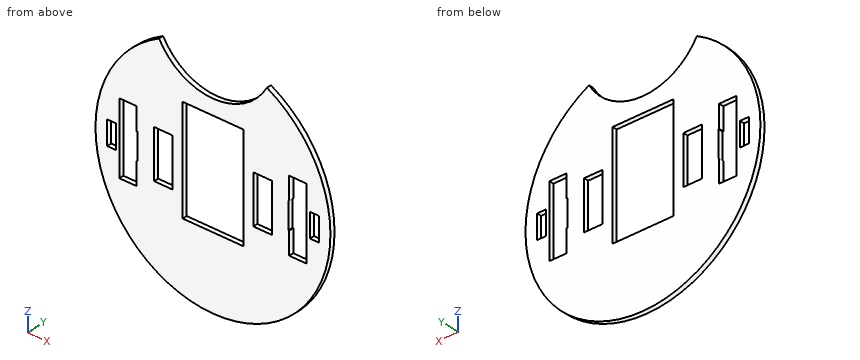
from build123d import *

# Parameters (mm, degrees)
BOSS_EXTRUDE1_DEPTH  = 2.9
SOLENOID_PLACEMENT_W = 37.4
SOLENOID_PLACEMENT_H = 63.8
CUT_EXTRUDE1_DEPTH   = 103.571487266
SKETCH2_W            = 10.76
SKETCH2_H            = 43.707605188
CUT_EXTRUDE2_DEPTH   = 103.571487266
SKETCH3_W            = 11.4
SKETCH3_H            = 29.6
CUT_EXTRUDE3_DEPTH   = 103.571487266
SKETCH5_W            = 5.5
SKETCH5_H            = 14.6
CUT_EXTRUDE4_DEPTH   = 103.571487266
SKETCH6_W            = 0.73
SKETCH6_H            = 16.225619988
CUT_EXTRUDE5_DEPTH   = 103.571487266


with BuildPart() as part:
    # Sketch1 → Boss-Extrude1 (new body)
    with BuildSketch(Plane(origin=(0, 0, 0), x_dir=(1, 0, 0), z_dir=(0, 1, 0))):
        with BuildLine():
            ThreePointArc((33.29110537, -64.404598464), (0, 72.5), (-33.29110537, -64.404598464))
            ThreePointArc((-33.29110537, -64.404598464), (0, -44.989799638), (33.29110537, -64.404598464))
        make_face()
    extrude(amount=BOSS_EXTRUDE1_DEPTH)

    # solenoid placement → Cut-Extrude1 (cut, through all)
    with BuildSketch(Plane(origin=(0, 2.9, 0), x_dir=(1, 0, 0), z_dir=(0, 1, 0))):
        with Locations((0, -3.8)):
            Rectangle(SOLENOID_PLACEMENT_W, SOLENOID_PLACEMENT_H)
    extrude(amount=-CUT_EXTRUDE1_DEPTH, mode=Mode.SUBTRACT)

    # Sketch2 → Cut-Extrude2 (cut, through all)
    with BuildSketch(Plane(origin=(0, 2.9, 0), x_dir=(1, 0, 0), z_dir=(0, 1, 0))):
        with Locations((52.42, 0)):
            Rectangle(SKETCH2_W, SKETCH2_H)
        with Locations((-52.42, 0)):
            Rectangle(SKETCH2_W, SKETCH2_H)
    extrude(amount=-CUT_EXTRUDE2_DEPTH, mode=Mode.SUBTRACT)

    # Sketch3 → Cut-Extrude3 (cut, through all)
    with BuildSketch(Plane(origin=(0, 2.9, 0), x_dir=(1, 0, 0), z_dir=(0, 1, 0))):
        with Locations((-30.61, 0)):
            Rectangle(SKETCH3_W, SKETCH3_H)
        with Locations((30.61, 0)):
            Rectangle(SKETCH3_W, SKETCH3_H)
    extrude(amount=-CUT_EXTRUDE3_DEPTH, mode=Mode.SUBTRACT)

    # Sketch5 → Cut-Extrude4 (cut, through all)
    with BuildSketch(Plane(origin=(0, 2.9, 0), x_dir=(1, 0, 0), z_dir=(0, 1, 0))):
        with Locations((-62.58, 0)):
            Rectangle(SKETCH5_W, SKETCH5_H)
        with Locations((62.58, 0)):
            Rectangle(SKETCH5_W, SKETCH5_H)
    extrude(amount=-CUT_EXTRUDE4_DEPTH, mode=Mode.SUBTRACT)

    # Sketch6 → Cut-Extrude5 (cut, through all)
    with BuildSketch(Plane(origin=(0, 2.9, 0), x_dir=(1, 0, 0), z_dir=(0, 1, 0))):
        with Locations((-46.975, 0)):
            Rectangle(SKETCH6_W, SKETCH6_H)
        with Locations((46.975, 0)):
            Rectangle(SKETCH6_W, SKETCH6_H)
    extrude(amount=-CUT_EXTRUDE5_DEPTH, mode=Mode.SUBTRACT)


solid = part.part
For this review, take the finished solid that the model builds, in its own axes (mm). Round coordinates to 2 decimals unless told otherwise and drop trailing zeros. Order: outer loops, then holes, each group sorted by start corner. A loop starts at its lowest first (then second) coordinate and runs counter-clockwise, first axis right, second up. Notation, with made-up numbers: (-10.5, 18) -> (20.5, 18) arc R26 ccw to (20.5, 41) -> close; hole circle Ø11 at (79, 37). An arc over 180 degrees is marked (long way). Put each result on its own line as item: value.
Q1. Add section C-C on z = 52. Write out the cut boundary in (x, y).
Check result:
outline: (-50.52, 0) -> (-22.07, 0) -> (-22.07, 2.9) -> (-50.52, 2.9) -> close; (22.07, 0) -> (50.52, 0) -> (50.52, 2.9) -> (22.07, 2.9) -> close
Q2. Insertion check: pin 1 Ø1.4 at (y, z) = (1.5, 19.5) entering from +X; pin 2 Ø0.9 at (y, z) = (1.5, 1) entering from +X; pin 3 Ø1.5 at (x, y) = (-28, 2.5) entering from +Z. Each pin has a flat end and moves straight along its axis. Give the tip position at first contact, or say it passes through.
Check result:
pin 1: x = 70.02
pin 2: x = 72.5
pin 3: z = 58.01
Q3. For probe 1 along X at (y, z) = (2.75, 19.5); probe 2 along X at (y, z) = (0.7, -17.5); probe 3 along Z at (x, y) = (55.5, 2), list the stretches that pass through material, from the lowest coordinate up. Write a range as [from, to].
Check result:
probe 1: [-69.83, -57.8], [-47.04, -18.7], [18.7, 47.04], [57.8, 69.83]
probe 2: [-70.36, -57.8], [-47.04, -18.7], [18.7, 47.04], [57.8, 70.36]
probe 3: [-46.65, -21.85], [21.85, 46.65]
Q4. Add section A-A on x = 0. Write out the cut boundary in (y, z), plus the area to 3 significant figures.
Check result:
outline: (0, -72.5) -> (2.9, -72.5) -> (2.9, -28.1) -> (0, -28.1) -> close; (0, 35.7) -> (2.9, 35.7) -> (2.9, 44.99) -> (0, 44.99) -> close
area: 156 mm2
Q5. Add section B-B on z = 0. State how many separate pieces and enclosed holes the cut face has, plus the area to 3 significant figures.
Check result:
separate pieces: 8
enclosed holes: 0
area: 149 mm2
